Here's how the part is built. I have some questions about the finished solid (model axes, mm). A direction names the side the tool comes from. Round coordinates to 2 decimals unless told otherwise and drop trailing zeros. Loops run counter-clockwise (first coordinate to the right, second up) from the corner with the lowest first, then second, coordinate; pieces in that order, holes last. Notation, with made-up numbers: M 24.25,9.5 L 61.25,9.5 A31 ccw 61.25,34.5 Z; hole C 8.5,84.25 d3. An arc over 180 degrees is marked long. Use a Markdown table: item, result.
from build123d import *

# Parameters (mm, degrees)
F0_W     = 74.0873217583
F0_H     = 72.1489936113
F1_DEPTH = 25.4
F2_R     = 4.445
F3_DEPTH = 25.4
F4_W     = 19.05
F4_H     = 38.1
F6_W     = 10.4351935416
F6_H     = 10.16
F8_SIZE  = 3.81
F9_R     = 2.54
F10_R    = 2.54


with BuildPart() as f1:
    # F0 (on Top) → F1 (new body)
    with BuildSketch(Plane.XY):
        Rectangle(F0_W, F0_H)
    extrude(amount=F1_DEPTH)

    # F2 (on face) → F3 (cut)
    with BuildSketch(Plane(origin=(0, 0, 0), x_dir=(1, 0, 0), z_dir=(0, 0, -1))):
        with Locations((27.5186608791, -26.5494968057)):
            Circle(F2_R)
        with Locations((27.5186608791, 26.5494968057)):
            Circle(F2_R)
        with Locations((-27.5186608791, 26.5494968057)):
            Circle(F2_R)
        with Locations((-27.5186608791, -26.5494968057)):
            Circle(F2_R)
    extrude(amount=-F3_DEPTH, mode=Mode.SUBTRACT)

    # F4 (on Front) → F5 (revolve)
    with BuildSketch(Plane.XZ):
        with Locations((-9.525, 44.45)):
            Rectangle(F4_W, F4_H)
    revolve(axis=Axis((0, 0, 44.45), (0, 0, -1)))

    # F6 (on Right) → F7 (revolve, cut)
    with BuildSketch(Plane.YZ):
        with Locations((17.8258673744, 43.18)):
            Rectangle(F6_W, F6_H)
    revolve(axis=Axis((0, 0, 63.5), (0, 0, -1)), mode=Mode.SUBTRACT)

    # F8
    f8_edges = [f1.edges().sort_by_distance(p)[0] for p in [
        (-37.043661, 0, 25.4),
        (0, -36.074497, 25.4),
        (37.043661, 0, 25.4),
        (0, 36.074497, 25.4),
    ]]
    chamfer(f8_edges, length=F8_SIZE)

    # F9
    f9_edges = [f1.edges().sort_by_distance(p)[0] for p in [
        (19.05, 0, 38.1),
        (19.05, 0, 48.26),
        (19.05, 0, 25.4),
    ]]
    fillet(f9_edges, radius=F9_R)

    # F10
    f10_edges = [f1.edges().sort_by_distance(p)[0] for p in [
        (19.05, 0, 63.5),
    ]]
    fillet(f10_edges, radius=F10_R)


solid = f1.part
1. For pin 1 Ø4 at (x, y) = (-19, -25.5) entering from +Z; pin 2 Ø10 at (x, z) = (-7.5, 34) entering from +Y; pin 3 Ø5 at (x, z) = (-27.5, 27) entering from -Y, each with a flat end and sliding along its axis, tell me the tip position at first contact or that it passes through.
Answer sheet:
| item | result |
|---|---|
| pin 1 | z = 25.4 |
| pin 2 | y = 18.89 |
| pin 3 | y = -33.16 |
2. I need wall thicknesses on probe 1 along X at (y, z) = (25, 22.5); probe 2 along Z at (x, y) = (-33, -10.5); probe 3 along Z at (x, y) = (-14.5, 1.5). Which ranges of each line are inside material? Lowest first, please. Write a range as from..to.
Answer sheet:
| item | result |
|---|---|
| probe 1 | -36.13..-31.68, -23.35..23.35, 31.68..36.13 |
| probe 2 | 0..25.4 |
| probe 3 | 0..38.1, 48.26..63.5 |
3. Which directions (+Z, -Z, +X, -X, +Y, -Y) give clear straight access to the entire face, cutting with the end or side of a thin tool? Please do faces 1 (the face through (-12.31, -2.73, 43.25)), 2 (the face through (-37.044, -1, 11)), 3 (the face through (15.12, -11.59, 31.8)).
Answer sheet:
| item | result |
|---|---|
| face 1 | none |
| face 2 | +Z, -Z, -X, +Y, -Y |
| face 3 | +Z |
4. Imagine slicing it at A-A, the plane x = 0. Write out the boundary of the cut face in (y, z), then the cut area to 3 significant figures.
Answer sheet:
| item | result |
|---|---|
| outline | M -36.07,0 L 36.07,0 L 36.07,21.59 L 32.26,25.4 L 21.59,25.4 A2.54 cw 19.05,27.94 L 19.05,35.56 A2.54 ccw 16.51,38.1 L 12.61,38.1 L 12.61,48.26 L 16.51,48.26 A2.54 ccw 19.05,50.8 L 19.05,60.96 A2.54 ccw 16.51,63.5 L -16.51,63.5 A2.54 ccw -19.05,60.96 L -19.05,50.8 A2.54 ccw -16.51,48.26 L -12.61,48.26 L -12.61,38.1 L -16.51,38.1 A2.54 ccw -19.05,35.56 L -19.05,27.94 A2.54 cw -21.59,25.4 L -32.26,25.4 L -36.07,21.59 Z |
| area | 3,130 mm2 |
5. We'd pull the mould along Y, two halves only. Please class faces 4 (the face through (0, 22, 25.4)), 5 (the face through (31.758, 25.214, 12.522)), 6 (the face through (29.57, -22.606, 12.522)), 7 (the face through (15.12, -11.59, 55.95)): +Y half, -Y half, draft (parallel to the pull), parting line (faces both ways), or undercut.
Answer sheet:
| item | result |
|---|---|
| face 4 | draft |
| face 5 | undercut |
| face 6 | undercut |
| face 7 | parting line |
6. Imagine slicing it at B-B, the plane y = 0. Write out the boundary of the cut face in (x, z).
Answer sheet:
| item | result |
|---|---|
| outline | M -37.04,0 L 37.04,0 L 37.04,21.59 L 33.23,25.4 L 21.59,25.4 A2.54 cw 19.05,27.94 L 19.05,35.56 A2.54 ccw 16.51,38.1 L 12.61,38.1 L 12.61,48.26 L 16.51,48.26 A2.54 ccw 19.05,50.8 L 19.05,60.96 A2.54 ccw 16.51,63.5 L -16.51,63.5 A2.54 ccw -19.05,60.96 L -19.05,50.8 A2.54 ccw -16.51,48.26 L -12.61,48.26 L -12.61,38.1 L -16.51,38.1 A2.54 ccw -19.05,35.56 L -19.05,27.94 A2.54 cw -21.59,25.4 L -33.23,25.4 L -37.04,21.59 Z |
7. Imagine slicing it at C-C, the plane z = 53. Write out the boundary of the cut face in (x, y), then the cut area to 3 significant figures.
Answer sheet:
| item | result |
|---|---|
| outline | C 0,0 d38.1 |
| area | 1,140 mm2 |
